from build123d import *

# Parameters (mm, degrees)
SKETCH_W        = 18.5
SKETCH_H        = 26
PAD_DEPTH       = 15
SKETCH001_W     = 12.5
SKETCH001_H     = 23
POCKET_DEPTH    = 15
SKETCH002_W     = 30
SKETCH002_H     = 7
POCKET001_DEPTH = 1
PAD001_DEPTH    = 15
SKETCH004_R     = 1.5
POCKET002_DEPTH = 15
SKETCH005_W     = 30
SKETCH005_H     = 7
POCKET003_DEPTH = 1
SKETCH006_W     = 30
SKETCH006_H     = 7
POCKET004_DEPTH = 2
SKETCH007_W     = 7
SKETCH007_H     = 7
POCKET005_DEPTH = 4
SKETCH008_R     = 3
POCKET006_DEPTH = 10
FILLET_R        = 5
FILLET001_R     = 3
FILLET002_R     = 1
FILLET003_R     = 2


with BuildPart() as part:
    # Sketch → Pad (new body)
    with BuildSketch(Plane.XY):
        with Locations((9.25, 13)):
            Rectangle(SKETCH_W, SKETCH_H)
    extrude(amount=PAD_DEPTH)

    # Sketch001 (on Face6 of Pad) → Pocket (cut)
    with BuildSketch(Plane.XY.offset(15)):
        with Locations((9.25, 11.5)):
            Rectangle(SKETCH001_W, SKETCH001_H)
    extrude(amount=-POCKET_DEPTH, mode=Mode.SUBTRACT)

    # Sketch002 (on Face6 of Pocket) → Pocket001 (cut)
    with BuildSketch(Plane(origin=(0, 26, 0), x_dir=(-1, 0, 0), z_dir=(0, 1, 0))):
        with Locations((-15, 7.5)):
            Rectangle(SKETCH002_W, SKETCH002_H)
    extrude(amount=-POCKET001_DEPTH, mode=Mode.SUBTRACT)

    # Sketch003 (on Face4 of Pocket001) → Pad001 (join)
    with BuildSketch(Plane.XY):
        Polygon((18.5, 13.821131), (18.5, 0.321131), (32, 0.321131), align=None)
    extrude(amount=PAD001_DEPTH)

    # Sketch004 (on Face19 of Pad001) → Pocket002 (cut)
    with BuildSketch(Plane(origin=(16.160565, 16.160566, 0), x_dir=(-0.707107, 0.707107, 0), z_dir=(0.707107, 0.707107, 0))):
        with Locations((-13, 7.5)):
            Circle(SKETCH004_R)
    extrude(amount=-POCKET002_DEPTH, mode=Mode.SUBTRACT)

    # Sketch005 (on Face5 of Pocket002) → Pocket003 (cut)
    with BuildSketch(Plane(origin=(0, 0, 0), x_dir=(0, -1, 0), z_dir=(-1, 0, 0))):
        with Locations((-15, 7.5)):
            Rectangle(SKETCH005_W, SKETCH005_H)
    extrude(amount=-POCKET003_DEPTH, mode=Mode.SUBTRACT)

    # Sketch006 (on Face13 of Pocket003) → Pocket004 (cut)
    with BuildSketch(Plane.YZ.offset(18.5)):
        with Locations((15, 7.5)):
            Rectangle(SKETCH006_W, SKETCH006_H)
    extrude(amount=-POCKET004_DEPTH, mode=Mode.SUBTRACT)

    # Sketch007 (on Face15 of Pocket004) → Pocket005 (cut)
    with BuildSketch(Plane(origin=(15.5, 0, 0), x_dir=(0, -1, 0), z_dir=(-1, 0, 0))):
        with Locations((-3.5, 7.5)):
            Rectangle(SKETCH007_W, SKETCH007_H)
    extrude(amount=-POCKET005_DEPTH, mode=Mode.SUBTRACT)

    # Sketch008 (on Face29 of Pocket005) → Pocket006 (cut)
    with BuildSketch(Plane(origin=(13.332138, 13.332138, 0), x_dir=(-0.707107, 0.707107, 0), z_dir=(0.707107, 0.707107, 0))):
        with Locations((-13, 7.5)):
            Circle(SKETCH008_R)
    extrude(amount=-POCKET006_DEPTH, mode=Mode.SUBTRACT)

    # Fillet
    fillet_edges = [part.edges().sort_by_distance(p)[0] for p in [
        (15.5, 23, 7.5),
        (3, 23, 7.5),
    ]]
    fillet(fillet_edges, radius=FILLET_R)

    # Fillet001
    fillet001_edges = [part.edges().sort_by_distance(p)[0] for p in [
        (0, 26, 13),
        (18.5, 26, 13),
        (18.5, 26, 2),
        (0, 26, 2),
        (1, 25, 7.5),
        (16.5, 25, 7.5),
    ]]
    fillet(fillet001_edges, radius=FILLET001_R)

    # Fillet002
    fillet002_edges = [part.edges().sort_by_distance(p)[0] for p in [
        (32, 0.321131, 7.5),
    ]]
    fillet(fillet002_edges, radius=FILLET002_R)

    # Fillet003
    fillet003_edges = [part.edges().sort_by_distance(p)[0] for p in [
        (30.509666, 0.938448, 15),
        (30.509666, 0.938448, 0),
    ]]
    fillet(fillet003_edges, radius=FILLET003_R)


solid = part.part
Work out the finished part from the listing and answer in its coordinate system (mm). A direction names the side the tool comes from. Round coordinates to 2 decimals unless told otherwise and drop trailing zeros. Write each loop counter-clockwise with the first axis right and the second up, starting at its lowest first coordinate (ties: lowest second). Pieces come first, ordered by that corner, then holes. Notation, with made-up numbers: (-11, 77.25) - (6, 77.25) arc R20 ccw to (6, 84.25) - close; hole circle Ø7 at (-20.75, 12). An arc over 180 degrees is marked (long way). Answer in a Markdown table with one row per item. Add a question column.
1. A cutting plane is placed at D-D, the plane z = 7. Determine the outline of the cut face in (x, y), and give its area (3 significant figures).
2. Given pin 1 (3 mm diameter, centred on x = 9, z = 11, fed in from -Y); pin 2 (2 mm diameter, centred on y = 14.5, z = 7, fed in from +X); pin 3 (9 mm diameter, centred on x = 26, z = 7.5, fed in from -Y), each flat-ended and moving along its own axis, determine where each tip first touches the part or whether it passes through.
3. A cutting plane is placed at C-C, the plane y = 11.5. Count the separate pieces of the cut face and the enclosed holes in it, and give its area (3 significant figures).
4. A cutting plane is placed at A-A, the plane z = 12.25. Determine the outline of the cut face in (x, y), and give its area (3 significant figures).
5. Find the intervals of material crossed by line 1 along X through (y, z) = (14.75, 10); line 2 along X through (y, z) = (15.25, 12); line 3 along X through (y, z) = (7.75, 5.25), in increasing order. Write a range as from..to.
6. The mould has two halves that part along Z. Classify faces 1 (the flat face through (17, 14, 4)), 2 (the cylindrical face through (23.965, 0.923, 0.57)), 3 (the cylindrical face through (1.86, 24.1, 7.55)), 4 (the flat face through (15.5, 11, 8)): +Z half, -Z half, draft (parallel to the pull), parting line (faces both ways), or undercut.
7. A cutting plane is placed at B-B, the plane x = 10. Determine the outline of the cut face in (y, z), and give its area (3 significant figures).
8. For faces 5 (the flat face through (1, 11, 8)), 6 (the flat face through (21.611, 5.053, 6.209)), 7 (the flat face through (9, 23, 8)), determine the directions among +Z, -Z, +X, -X, +Y, -Y from which every point of the face is accessible in a straight line to the end or side of a thin tool.
Worked out:
| question | item | result |
|---|---|---|
| 1 | outline | (1, 0) - (3, 0) - (3, 18) arc R5 cw to (8, 23) - (10.5, 23) arc R5 cw to (15.5, 18) - (15.5, 7) - (16.5, 7) - (16.5, 22) arc R3 ccw to (13.5, 25) - (4, 25) arc R3 ccw to (1, 22) - close; (18.5, 7) - (19.5, 7) - (19.5, 5.3) - (20.43, 6.23) - (21.52, 5.14) - (24.35, 7.97) - (18.5, 13.82) - close; (22.89, 0.32) - (29.59, 0.32) arc R1 ccw to (30.29, 2.03) - (26.35, 5.97) - (23.52, 3.14) - (24.62, 2.05) - close |
| 1 | area | 152 mm^2 |
| 2 | pin 1 | y = 22.97 |
| 2 | pin 2 | x = 18.82 |
| 2 | pin 3 | y = 0.32 |
| 3 | separate pieces | 2 |
| 3 | enclosed holes | 1 |
| 3 | area | 101 mm^2 |
| 4 | outline | (0, 0) - (3, 0) - (3, 18) arc R5 cw to (8, 23) - (10.5, 23) arc R5 cw to (15.5, 18) - (15.5, 0) - (18.5, 0) - (18.5, 0.32) - (29.59, 0.32) arc R1 ccw to (30.29, 2.03) - (18.5, 13.82) - (18.5, 23) arc R3 ccw to (15.5, 26) - (3, 26) arc R3 ccw to (0, 23) - close |
| 4 | area | 290 mm^2 |
| 5 | line 1 | 1..3, 15.5..16.5 |
| 5 | line 2 | 0..3, 15.5..18.5 |
| 5 | line 3 | 1..3, 15.5..16.5, 18.5..24.57 |
| 6 | face 1 | undercut |
| 6 | face 2 | -Z half |
| 6 | face 3 | undercut |
| 6 | face 4 | draft |
| 7 | outline | (23, 0) - (26, 0) - (26, 4) - (25, 4) - (25, 11) - (26, 11) - (26, 15) - (23, 15) - close |
| 7 | area | 38.0 mm^2 |
| 8 | face 5 | -X, +Y, -Y |
| 8 | face 6 | none |
| 8 | face 7 | +Z, -Z, -Y |
